Geometry check sheet. Reference: the model listing, model coordinates, mm. Face numbers are marked on the shaded views. A direction names the side the tool comes from. Round coordinates to 2 decimals unless told otherwise and drop trailing zeros. Write each loop counter-clockwise with the first axis right and the second up, starting at its lowest first coordinate (ties: lowest second). Pieces come first, ordered by that corner, then holes. Notation, with made-up numbers: (21, 70) -> (33, 70) arc R3 ccw to (33, 75) -> close; hole circle Ø4 at (53, 18.5). An arc over 180 degrees is marked (long way). Use a Markdown table: item, result.
```python
from build123d import *

# Parameters (mm, degrees)
F0_W     = 136.9314
F0_H     = 120.65
F2_DEPTH = 5.08
F1_W     = 85.725
F1_H     = 55.5625
F1_W_2   = 68.58
F1_H_2   = 53.34
F1_R     = 1.5875
F3_DEPTH = 3.175


# Not quite as in the source:
# - the program builds the solid bodies; features that only make, move or delete a surface that nothing else refers to are left out


with BuildPart() as f2:
    # F0 (on Top) → F2 (new body)
    with BuildSketch(Plane.XY):
        Rectangle(F0_W, F0_H)
    extrude(amount=F2_DEPTH)

    # F1 (on Top) → F3 (cut)
    with BuildSketch(Plane.XY):
        with Locations((17.2909619287, 28.73375)):
            Rectangle(F1_W, F1_H)
        with Locations((25.8121827105, -29.845)):
            Rectangle(F1_W_2, F1_H_2)
        with Locations((5.4921827105, -53.975)):
            Circle(F1_R, mode=Mode.SUBTRACT)
        with Locations((6.7621827105, -5.715)):
            Circle(F1_R, mode=Mode.SUBTRACT)
        with Locations((57.5621827105, -48.895)):
            Circle(F1_R, mode=Mode.SUBTRACT)
        with Locations((57.5621827105, -20.955)):
            Circle(F1_R, mode=Mode.SUBTRACT)
    extrude(amount=F3_DEPTH, mode=Mode.SUBTRACT)


solid = f2.part
```
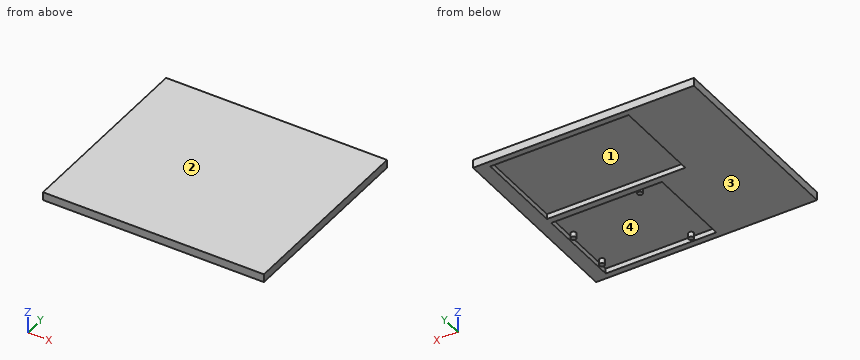
(1) Section check D-D on y = 23.5. Record the cut outline in (x, z) (3 decimals), plus the area to 3 significant figures.
A:
| item | result |
|---|---|
| outline | (-68.466, 0) -> (-25.572, 0) -> (-25.572, 3.175) -> (60.153, 3.175) -> (60.153, 0) -> (68.466, 0) -> (68.466, 5.08) -> (-68.466, 5.08) -> close |
| area | 423 mm2 |
(2) Section check C-C on y = -15.5. Record the cut outline in (x, z) (3 decimals).
A:
| item | result |
|---|---|
| outline | (-68.466, 0) -> (-8.478, 0) -> (-8.478, 3.175) -> (60.102, 3.175) -> (60.102, 0) -> (68.466, 0) -> (68.466, 5.08) -> (-68.466, 5.08) -> close |
(3) Section check A-A on z = 2.4. Record the cut outline in (x, y) (1 decimal).
A:
| item | result |
|---|---|
| outline | (-68.5, -60.3) -> (68.5, -60.3) -> (68.5, 60.3) -> (-68.5, 60.3) -> close; circle Ø3.2 at (5.5, -54); circle Ø3.2 at (6.8, -5.7); circle Ø3.2 at (57.6, -48.9); circle Ø3.2 at (57.6, -21); hole (-25.6, 1) -> (60.2, 1) -> (60.2, 56.5) -> (-25.6, 56.5) -> close; hole (-8.5, -56.5) -> (60.1, -56.5) -> (60.1, -3.2) -> (-8.5, -3.2) -> close |
(4) Section check B-B on x = 30. Record the cut outline in (y, z) (1 decimal), plus the area to 3 significant figures.
A:
| item | result |
|---|---|
| outline | (-60.3, 0) -> (-56.5, 0) -> (-56.5, 3.2) -> (-3.2, 3.2) -> (-3.2, 0) -> (1, 0) -> (1, 3.2) -> (56.5, 3.2) -> (56.5, 0) -> (60.3, 0) -> (60.3, 5.1) -> (-60.3, 5.1) -> close |
| area | 267 mm2 |
(5) Release check for a two-part mould opening along X. For the marked faces 1 and 2 record: +X half, -X half, draft (parallel to the pull), parting line (faces both ways), or undercut.
A:
| item | result |
|---|---|
| face 1 | undercut |
| face 2 | draft |
(6) Access from +Z, -Z, +X, -X, +Y, -Y to the whole of each face (thin tool, end or side, straight path). Record for the marked faces 3 and 4.
A:
| item | result |
|---|---|
| face 3 | -Z, +X, -X, +Y, -Y |
| face 4 | -Z |
(7) Gauge pin test, flat end, axial feed: pin 1 Ø3 at (x, y) = (5, -10.5) entering from -Z (3 decimals). Record the tip position at first contact, or that the pin passes through.
A:
| item | result |
|---|---|
| pin 1 | stops at z = 3.175 |
(8) Thickness scan on line 1 (Y direction, x = -7.5, z = 0.85) (1 decimal); line 2 (X direction, y = -37.5, z = 2.95); line 3 (Y direction, x = 6, z = 1.85) (1 decimal). Record the ranges inside material, lowest first.
A:
| item | result |
|---|---|
| line 1 | y = -60.3 to -56.5, -3.2 to 1, 56.5 to 60.3 |
| line 2 | x = -68.47 to -8.48, 60.1 to 68.47 |
| line 3 | y = -60.3 to -56.5, -55.5 to -52.5, -7.1 to -4.3, -3.2 to 1, 56.5 to 60.3 |
